Autodesk Inventor part; units mm, degrees
ref_plane "Work Plane2" through (-44.45, 19.05, 25.4) normal (0, 0, 1) x (1, 0, 0)
ref_plane "Work Plane3" through (-48.5775, -83.82, 6.35) normal (0, 0, 1) x (1, 0, 0)
ref_plane "Work Plane4" through (-45.085, 18.415, 12.9) normal (0, 0, 1) x (1, 0, 0)
ref_plane "Work Plane1" through (0, 0, 0.2032) normal (0, 0, 1) x (1, 0, 0)
sketch "Sketch1" plane through (0, 0, 0.2032) normal (0, 0, 1) x (1, 0, 0)
  circle A0 centre (-38.1, 25.4) radius 6.35 construction
  circle A1 centre (-38.1, -25.4) radius 6.35
  circle A2 centre (-38.1, 25.4) radius 6.35 construction
  circle A3 centre (-38.1, 25.4) radius 6.75
  circle A4 centre (-38.1, 25.4) radius 19.05 construction
  circle A5 centre (-38.1, 25.4) radius 19.05
  point P0 (0, 0)
  dimension "d0" = 0.4
ref_plane "Work Plane2" through (-44.45, 19.05, 25.4) normal (0, 0, 1) x (1, 0, 0)
ref_plane "Work Plane3" through (-48.5775, -83.82, 6.35) normal (0, 0, 1) x (1, 0, 0)
extrude "Extrusion1" add sketch "Sketch1" along normal up to surface (6.1468 mm away) contours A5
sketch "Sketch2" plane through (-38.1, 25.4, 6.35) normal (0, 0, 1) x (1, 0, 0)
  circle A0 centre (0, 0) radius 6.75
  circle A1 centre (0, 0) radius 19.05
  circle A2 centre (0, 0) radius 16.51
  point P0 (38.1, -25.4)
  dimension "d3" = 2.54
ref_plane "Work Plane4" through (-45.085, 18.415, 12.9) normal (0, 0, 1) x (1, 0, 0)
extrude "Extrusion2" add sketch "Sketch2" along normal up to surface (6.55 mm away) contours A2
sketch "Sketch3" plane through (-38.1, 25.4, 12.9) normal (0, 0, 1) x (1, 0, 0)
  circle A0 centre (0, 0) radius 6.75
  circle A1 centre (0, 0) radius 16.51
  circle A2 centre (0, 0) radius 19.05
  circle A3 centre (0, 0) radius 16.51
  circle A4 centre (0, 0) radius 19.05
  point P0 (38.1, -25.4)
ref_plane "Work Plane5" through (-44.45, 19.05, 19.25) normal (0, 0, 1) x (1, 0, 0)
ref_plane "Work Plane6" through (-44.45, 19.05, 19.25) normal (0, 0, 1) x (1, 0, 0)
extrude "Extrusion3" add sketch "Sketch3" along normal up to surface (6.35 mm away) contours A1 | A2
properties part number "Cart Wheel"
Can you work these out from the model? Positions are in its coordinate system, mm. A direction names the side the tool comes from. Coordinates: 2 decimals unless noted, no trailing zeros. Loops run counter-clockwise (first coordinate to the right, second up) from the corner with the lowest first, then second, coordinate; pieces in that order, holes last. Notation, with made-up numbers: M 52,77.5 L 103,77.5 A13 cw 103,94.5 Z; hole C 23.5,65.25 d7. An arc over 180 degrees is marked long. Answer as CSV lines item,"result". Start each with the question number.
1. For faces 1 (the face through (-19.93, 19.68, 16.03)), 2 (the face through (-44, 41, 12.9)), which set-ups out of +Z, -Z, +X, -X, +Y, -Y let a thin tool reach every point of the face, with its end or its side?
2. Thinking about a two-plate mould opening in Y: for faces 3 (the face through (-44.843, 25.103, 9.593)), 4 (the face through (-19.93, 19.68, 3.23)), 5 (the face through (-38, 17, 0.203)), which applies, +Y half, -Y half, draft (parallel to the pull), parting line (faces both ways), or undercut?
3. If I drill on probe 1 along Y at (x, z) = (-38.1, 11.75); probe 2 along Z at (x, y) = (-50, 13.5); probe 3 along Y at (x, z) = (-38.1, 15), over which ranges is the centre line in solid material (lowest first)? Write a range as [from, to].
4. For pin 1 Ø19 at (x, y) = (-42.5, 24) entering from +Z; pin 2 Ø8 at (x, z) = (-46, 7) entering from +Y; pin 3 Ø5 at (y, z) = (39.5, 9.5) entering from +X; pin 4 Ø8 at (y, z) = (33, 7) entering from -X, each with a flat end and sliding along its axis, tell me the tip position at first contact or that it passes through.
5. Suppose I cut it at D-D, the plane y = 13.5. List the corners of the cut face in (x, z) for me, plus the area to 3 significant figures.
6. Suppose I cut it at A-A, the plane x = -38.1. List the corners of the cut face in (y, z) for me, plus the area to 3 significant figures.
7. Suppose I cut it at C-C, the plane z = 7.25. List the corners of the cut face in (x, y) for me, plus the area to 3 significant figures.
8. Suppose I cut it at B-B, the plane y = 25.4. List the corners of the cut face in (x, z) for me, plus the area to 3 significant figures.
Output:
1,face 1,"+Z, -Z"
1,face 2,"none"
2,face 3,"undercut"
2,face 4,"parting line"
2,face 5,"draft"
3,probe 1,"y = [8.89, 18.65], [32.15, 41.91]"
3,probe 2,"z = [0.2, 6.35], [12.9, 19.25]"
3,probe 3,"y = [6.35, 18.65], [32.15, 44.45]"
4,pin 1,"stops at z = 19.25"
4,pin 2,"stops at y = 44.04"
4,pin 3,"stops at x = -26.35"
4,pin 4,"stops at x = -56.8"
5,outline,"M -52.98,0.2 L -23.22,0.2 L -23.22,6.35 L -26.66,6.35 L -26.66,12.9 L -23.22,12.9 L -23.22,19.25 L -52.98,19.25 L -52.98,12.9 L -49.54,12.9 L -49.54,6.35 L -52.98,6.35 Z"
5,area,"522 mm^2"
6,outline,"M 6.35,0.2 L 18.65,0.2 L 18.65,19.25 L 6.35,19.25 L 6.35,12.9 L 8.89,12.9 L 8.89,6.35 L 6.35,6.35 Z; M 32.15,0.2 L 44.45,0.2 L 44.45,6.35 L 41.91,6.35 L 41.91,12.9 L 44.45,12.9 L 44.45,19.25 L 32.15,19.25 Z"
6,area,"435 mm^2"
7,outline,"C -38.1,25.4 d33.02; hole C -38.1,25.4 d13.5"
7,area,"713 mm^2"
8,outline,"M -57.15,0.2 L -44.85,0.2 L -44.85,19.25 L -57.15,19.25 L -57.15,12.9 L -54.61,12.9 L -54.61,6.35 L -57.15,6.35 Z; M -31.35,0.2 L -19.05,0.2 L -19.05,6.35 L -21.59,6.35 L -21.59,12.9 L -19.05,12.9 L -19.05,19.25 L -31.35,19.25 Z"
8,area,"435 mm^2"
